Could you check a few things on this model? Use its own coordinates, in mm. A direction names the side the tool comes from. Give positions to 0.01 mm unless a question says otherwise; leave off trailing zeros. Write each loop counter-clockwise with the first axis right and the second up, starting at its lowest first coordinate (ties: lowest second). Pieces come first, ordered by that corner, then holes. Notation, with made-up numbers: (72.25, 29) - (88.25, 29) arc R34 ccw to (88.25, 63) - close; hole circle Ø9 at (-3.5, -28.75). An arc over 180 degrees is marked (long way). Answer as CSV lines item,"result". Start each with the question number.
Q1. Imagine slicing it at A-A on z = 6.25. List the corners of the cut face in (x, y) for me, and give its area (3 significant figures).
Q2. On a 3-axis mill with a long thin cutter (end or side, diameter ignored), from which of +Z, -Z, +X, -X, +Y, -Y can I reach the whole of each face in a straight line? I mean faces 1 (the face through (1, -0.75, 13)), 2 (the face through (-1, 1, 14)). Say none if no direction works.
Q3. Will these pins go through, and if not, where does the flat tip stop? pin 1 Ø4 at (x, y) = (-1, -2) entering from -Z; pin 2 Ø1.2 at (x, y) = (0.5, 0) entering from +Z; pin 3 Ø0.7 at (x, z) = (1.5, 11) entering from -Y; pin 4 Ø2 at (x, y) = (-3.5, 4) entering from -Z.
Q4. We'd pull the mould along Y, two halves only. Please class faces 3 (the face through (-1.914, -0.01, 11.976)), 4 (the face through (3, 4, 11)), 5 (the face through (0, 0, 0)): pulls with the +Y half, pulls with the -Y half, needs draft (parallel to the pull), parting line crosses it, or undercut.
Q5. If I drill on line 1 along Y through (x, z) = (0, 1.25); line 2 along Y through (x, z) = (0, 11); line 3 along X through (y, z) = (1.25, 1.5), over which ranges is the centre line in solid material (lowest first)?
```python
from build123d import *

# Parameters (mm, degrees)
SZKIC1_R                        = 3.5
DODANIE_WYCI_GNI_CIE1_DEPTH     = 10
SZKIC3_R                        = 5
DODANIE_WYCI_GNI_CIE2_DEPTH     = 4
SFAZOWANIE2_SIZE                = 2
SFAZOWANIE2_SIZE2               = 0.5
ZAOKR_GLENIE1_R                 = 1.5
ZAOKR_GLENIE2_R                 = 3
ZAOKR_GLENIE3_R                 = 0.5
WYTNIJ_WYCI_GNI_CIE1_DEPTH      = 0.75
WYTNIJ_WYCI_GNI_CIE1_DEPTH_BACK = 0.75
WYTNIJ_WYCI_GNI_CIE2_DEPTH      = 0.75
WYTNIJ_WYCI_GNI_CIE2_DEPTH_BACK = 0.75


with BuildPart() as part:
    # Szkic1 → Dodanie-wyciągnięcie1 (new body)
    with BuildSketch(Plane.XY):
        Circle(SZKIC1_R)
    extrude(amount=DODANIE_WYCI_GNI_CIE1_DEPTH)

    # Szkic3 → Dodanie-wyciągnięcie2 (add)
    with BuildSketch(Plane.XY.offset(10)):
        Circle(SZKIC3_R)
    extrude(amount=DODANIE_WYCI_GNI_CIE2_DEPTH)

    # Sfazowanie2
    sfazowanie2_edges = [part.edges().sort_by_distance(p)[0] for p in [
        (-5, 0, 14),
    ]]
    sfazowanie2_side = [part.faces().sort_by_distance(p)[0] for p in [
        (-5, 0, 12),
    ]]
    chamfer(sfazowanie2_edges, length=SFAZOWANIE2_SIZE, length2=SFAZOWANIE2_SIZE2, reference=sfazowanie2_side[0])

    # Zaokrąglenie1
    zaokr_glenie1_edges = [part.edges().sort_by_distance(p)[0] for p in [
        (-4.5, 0, 14),
    ]]
    fillet(zaokr_glenie1_edges, radius=ZAOKR_GLENIE1_R)

    # Zaokrąglenie2
    zaokr_glenie2_edges = [part.edges().sort_by_distance(p)[0] for p in [
        (-5, 0, 12),
    ]]
    fillet(zaokr_glenie2_edges, radius=ZAOKR_GLENIE2_R)

    # Zaokrąglenie3
    zaokr_glenie3_edges = [part.edges().sort_by_distance(p)[0] for p in [
        (-3.5, 0, 10),
    ]]
    fillet(zaokr_glenie3_edges, radius=ZAOKR_GLENIE3_R)

    # Szkic4 → Wytnij-wyciągnięcie1 (cut, two sides: drawn at the far end of the back side and taken through both)
    with BuildSketch(Plane(origin=(0, 0, 0), x_dir=(1, 0, 0), z_dir=(0, 1, 0)).offset(-WYTNIJ_WYCI_GNI_CIE1_DEPTH_BACK)):
        Polygon((3.045898371, -14), (-3.045898371, -14), (-0.25, -9), (0, -9), (0.25, -9), align=None)
    extrude(amount=WYTNIJ_WYCI_GNI_CIE1_DEPTH + WYTNIJ_WYCI_GNI_CIE1_DEPTH_BACK, mode=Mode.SUBTRACT)

    # Szkic5 → Wytnij-wyciągnięcie2 (cut, two sides: drawn at the far end of the back side and taken through both)
    with BuildSketch(Plane(origin=(0, 0, 0), x_dir=(0, 0, -1), z_dir=(1, 0, 0)).offset(-WYTNIJ_WYCI_GNI_CIE2_DEPTH_BACK)):
        Polygon((-9, 0), (-9, 0.25), (-14, 3.05), (-14, -3.05), (-9, -0.25), align=None)
    extrude(amount=WYTNIJ_WYCI_GNI_CIE2_DEPTH + WYTNIJ_WYCI_GNI_CIE2_DEPTH_BACK, mode=Mode.SUBTRACT)


solid = part.part
```
Conclusion:
1,outline,"circle Ø7 at (0, 0)"
1,area,"38.5 mm^2"
2,face 1,"+Z"
2,face 2,"+Z, +X, -X, +Y, -Y"
3,pin 1,"z = 0"
3,pin 2,"z = 10.52"
3,pin 3,"y = -4.87"
3,pin 4,"z = 10"
4,face 3,"undercut"
4,face 4,"parting line crosses it"
4,face 5,"needs draft"
5,line 1,"-3.5 to 3.5"
5,line 2,"-5 to -1.37, 1.37 to 5"
5,line 3,"-3.27 to 3.27"
